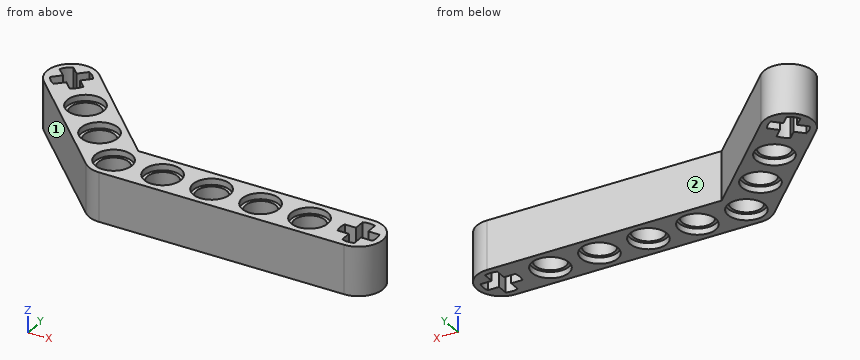
Autodesk Inventor part; units mm, degrees
ref_plane "YZ Plane" through (0, 0, 0) normal (1, 0, 0) x (0, 1, 0)
ref_plane "XZ Plane" through (0, 0, 0) normal (0, 1, 0) x (-1, 0, 0)
ref_plane "XY Plane" through (0, 0, 0) normal (0, 0, 1) x (1, 0, 0)
sketch "Sketch1" plane through (0, 0, 0) normal (0, 0, 1) x (1, 0, 0)
  arc A0 (-54.1421, 19.799) -> (-59.799, 14.1421) centre (-56.9706, 16.9706) ccw
  arc A1 (0, -4) -> (0, 4) centre (0, 0) ccw
  line L0 (-42.8284, -2.8284) -> (-59.799, 14.1421)
  line L1 (-38.3431, 4) -> (-54.1421, 19.799)
  line L2 (-75.9529, 0) -> (17.3255, 0)
  line L3 (0, -9.663) -> (0, 28.0092)
  line L4 (0, -4) -> (-40, -4)
  line L5 (0, 4) -> (-38.3431, 4)
  arc A2 (-42.8284, -2.8284) -> (-40, -4) centre (-40, 0) ccw
  dimension "d13" = 4
  dimension "d15" = 0
  dimension "d16" = 0
  dimension "d25" = 4
  dimension "d27" = 135
  dimension "d29" = 40
  dimension "d35" = 135
  dimension "d36" = 4
  dimension "d37" = 24
  dimension "d142" = 24
extrude "Extrusion1" add sketch "Sketch1" along normal blind 8
sketch "Sketch2" plane through (0, 0, 8) normal (0, 0, 1) x (1, 0, 0)
  arc A0 (-54.1421, 19.799) -> (-59.799, 14.1421) centre (-56.9706, 16.9706) ccw
  line L0 (-42.8284, -2.8284) -> (-59.799, 14.1421)
  arc A1 (-58.2635, 19.6777) -> (-59.6777, 18.2635) centre (-56.9706, 16.9706) ccw
  arc A2 (-59.6777, 15.6777) -> (-58.2635, 14.2635) centre (-56.9706, 16.9706) ccw
  arc A3 (-55.6777, 14.2635) -> (-54.2635, 15.6777) centre (-56.9706, 16.9706) ccw
  arc A4 (-54.2635, 18.2635) -> (-55.6777, 19.6777) centre (-56.9706, 16.9706) ccw
  line L1 (-54.2635, 18.2635) -> (-55.5563, 16.9706)
  line L2 (-56.9706, 15.5563) -> (-58.2635, 14.2635)
  line L3 (-59.6777, 18.2635) -> (-58.3848, 16.9706)
  line L4 (-56.9706, 15.5563) -> (-55.6777, 14.2635)
  line L5 (-55.6777, 19.6777) -> (-56.9706, 18.3848)
  line L6 (-58.3848, 16.9706) -> (-59.6777, 15.6777)
  line L7 (-58.2635, 19.6777) -> (-56.9706, 18.3848)
  line L8 (-55.5563, 16.9706) -> (-54.2635, 15.6777)
  dimension "d46" = 3
  dimension "d47" = 3
  dimension "d48" = 3
  dimension "d49" = 3
  dimension "d50" = 2
  dimension "d51" = 2
  dimension "d52" = 2
  dimension "d53" = 2
  dimension "d54" = 1
  dimension "d55" = 1
  dimension "d56" = 1
  dimension "d57" = 1
  dimension "d58" = 90
  dimension "d59" = 90
  dimension "d60" = 90
  dimension "d61" = 90
extrude "Extrusion2" cut sketch "Sketch2" against normal through all
sketch "Sketch3" plane through (0, 0, 8) normal (0, 0, 1) x (1, 0, 0)
  arc A0 (0, -4) -> (0, 4) centre (0, 0) ccw
  arc A1 (1, 2.8284) -> (-1, 2.8284) centre (0, 0) ccw
  arc A2 (-2.8284, 1) -> (-2.8284, -1) centre (0, 0) ccw
  arc A3 (-1, -2.8284) -> (1, -2.8284) centre (0, 0) ccw
  arc A4 (2.8284, -1) -> (2.8284, 1) centre (0, 0) ccw
  line L0 (-2.8284, -1) -> (-1, -1)
  line L1 (1, -1) -> (2.8284, -1)
  line L2 (-1, -2.8284) -> (-1, -1)
  line L3 (-1, 1) -> (-1, 2.8284)
  line L4 (-2.8284, 1) -> (-1, 1)
  line L5 (1, 1) -> (2.8284, 1)
  line L6 (1, -2.8284) -> (1, -1)
  line L7 (1, 1) -> (1, 2.8284)
  dimension "d65" = 3
  dimension "d66" = 3
  dimension "d67" = 3
  dimension "d68" = 3
  dimension "d69" = 2
  dimension "d70" = 2
  dimension "d71" = 2
  dimension "d72" = 2
  dimension "d73" = 90
  dimension "d74" = 90
  dimension "d75" = 90
  dimension "d76" = 1
  dimension "d77" = 1
  dimension "d78" = 1
  dimension "d79" = 1
  dimension "d80" = 2.8284
extrude "Extrusion3" cut sketch "Sketch3" against normal through all
sketch "Sketch10" plane through (0, 0, 8) normal (0, 0, 1) x (1, 0, 0)
  circle A0 centre (-8, 0) radius 2.5
  line L0 (-73.9647, 0) -> (16.9941, 0)
  line L1 (0, -21.6115) -> (0, 28.0676)
  circle A1 centre (-16, 0) radius 2.5
  circle A2 centre (-24, 0) radius 2.5
  circle A3 centre (-32, 0) radius 2.5
  circle A4 centre (-40, 0) radius 2.5
  point P0 (0, 0)
  dimension "d143" = 5
  dimension "d144" = 8
  dimension "d145" = 0
  dimension "d150" = 8
extrude "Extrusion10" cut sketch "Sketch10" against normal through all
sketch "Sketch11" plane through (0, 0, 8) normal (0, 0, 1) x (1, 0, 0)
  circle A0 centre (-45.6569, 5.6569) radius 2.5
  line L0 (-73.9647, 0) -> (16.9941, 0)
  line L1 (0, -8.9941) -> (0, 25.9647)
  line L2 (-54.1421, 19.799) -> (-38.3431, 4)
  circle A1 centre (-40, 0) radius 2.5
  circle A2 centre (-51.3137, 11.3137) radius 2.5
  point P0 (0, 0)
  dimension "d155" = 5
  dimension "d157" = 4
  dimension "d158" = 8
  dimension "d161" = 8
extrude "Extrusion11" cut sketch "Sketch11" against normal through all contours A0 | A2
sketch "Sketch12" plane through (0, 0, 8) normal (0, 0, 1) x (1, 0, 0)
  circle A0 centre (-8, 0) radius 2.5
  circle A1 centre (-8, 0) radius 3
  line L0 (-73.9647, 0) -> (16.9941, 0)
  circle A2 centre (-16, 0) radius 3
  circle A3 centre (-24, 0) radius 3
  circle A4 centre (-32, 0) radius 3
  circle A5 centre (-40, 0) radius 3
  point P0 (0, 0)
  dimension "d168" = 6
  dimension "d171" = 8
extrude "Extrusion12" cut sketch "Sketch12" against normal blind 1
sketch "Sketch13" plane through (0, 0, 8) normal (0, 0, 1) x (1, 0, 0)
  circle A0 centre (-45.6569, 5.6569) radius 2.5
  circle A1 centre (-51.3137, 11.3137) radius 2.5
  circle A2 centre (-51.3137, 11.3137) radius 3
  circle A3 centre (-45.6569, 5.6569) radius 3
  point P0 (0, 0)
  dimension "d178" = 6
  dimension "d179" = 6
extrude "Extrusion13" cut sketch "Sketch13" against normal blind 1 contours A0 | A1 | A2 | A3
sketch "Sketch14" plane through (0, 0, 0) normal (0, 0, -1) x (-1, 0, 0)
  circle A0 centre (8, 0) radius 2.5
  circle A1 centre (51.3137, 11.3137) radius 2.5
  circle A2 centre (45.6569, 5.6569) radius 2.5
  circle A3 centre (45.6569, 5.6569) radius 3
  circle A4 centre (51.3137, 11.3137) radius 3
  circle A5 centre (8, 0) radius 3
  circle A6 centre (8, 0) radius 3
  line L0 (73.9647, 0) -> (-16.9941, 0)
  line L1 (0, -4) -> (40, -4)
  circle A7 centre (16, 0) radius 3
  circle A8 centre (24, 0) radius 3
  circle A9 centre (32, 0) radius 3
  circle A10 centre (40, 0) radius 3
  point P0 (0, 0)
  dimension "d182" = 6
  dimension "d183" = 6
  dimension "d184" = 6
  dimension "d187" = 8
extrude "Extrusion14" cut sketch "Sketch14" against normal blind 1 contours L0 A0 | L0 A5 A0 | A0 L0 A5 | A0 L0 | A10 L0 | L0 A10 | A9 L0 | L0 A9 | A8 L0 | L0 A8 | A7 L0 | L0 A7 | A1 | A2 | A3 | A4
properties part number "9M Beam A 4X6"
Read the model definition and answer for the solid it produces. Units are mm, in the model's axes. Face numbers are marked on the shaded views. A direction names the side the tool comes from. Round coordinates to 2 decimals unless told otherwise and drop trailing zeros. Write each loop counter-clockwise with the first axis right and the second up, starting at its lowest first coordinate (ties: lowest second). Pieces come first, ordered by that corner, then holes. Notation, with made-up numbers: (43.25, -7) -> (101.25, -7) arc R14 cw to (101.25, 11) -> close; hole circle Ø4 at (69.25, 78.25). An arc over 180 degrees is marked (long way). Answer in a Markdown table with one row per item. Add a question column.
1) Find section B-B, the plane y = 0. State how many separate pieces and enclosed holes the cut face has, and give its area (3 significant figures).
2) Find section A-A, the plane x = -24. Determine the outline of the cut face in (y, z).
3) Which of the six approach directions +Z, -Z, +X, -X, +Y, -Y give full straight-line access (tool end or side, diameter ignored) to the marked faces 1 and 2?
4) Consider line 1 (Y direction, x = -8, z = 0.45); line 2 (Y direction, x = -40.5, z = 7.5); line 3 (X direction, y = 6, z = 3.5). Determine where each line is inside the solid, lowest interval first.
5) Given P1, Ø3, axis at x = -50.5, y = 11, coming from the -Z side; P2, Ø1.5, axis at y = -2, z = 4, coming from the +X side; P3, Ø4, axis at y = 14, z = 7, coming from the -X side; P4, Ø2, axis at y = 2, z = 3, coming from the -X side, each flat-ended and moving along its own axis, determine where each tip first touches the part or whether it passes through.
Findings below:
| question | item | result |
|---|---|---|
| 1 | separate pieces | 7 |
| 1 | enclosed holes | 0 |
| 1 | area | 139 mm² |
| 2 | outline | (-4, 0) -> (-3, 0) -> (-3, 1) -> (-2.5, 1) -> (-2.5, 7) -> (-3, 7) -> (-3, 8) -> (-4, 8) -> close; (2.5, 1) -> (3, 1) -> (3, 0) -> (4, 0) -> (4, 8) -> (3, 8) -> (3, 7) -> (2.5, 7) -> close |
| 3 | face 1 | +Z, -Z, -X, -Y |
| 3 | face 2 | +Z, -Z, +X, +Y |
| 4 | line 1 | -4 to -3, 3 to 4 |
| 4 | line 2 | -3.97 to -2.96, 2.96 to 6.16 |
| 4 | line 3 | -51.66 to -48.13, -43.18 to -40.34 |
| 5 | P1 | through |
| 5 | P2 | x = 3.8 |
| 5 | P3 | x = -60.85 |
| 5 | P4 | x = -48.66 |
